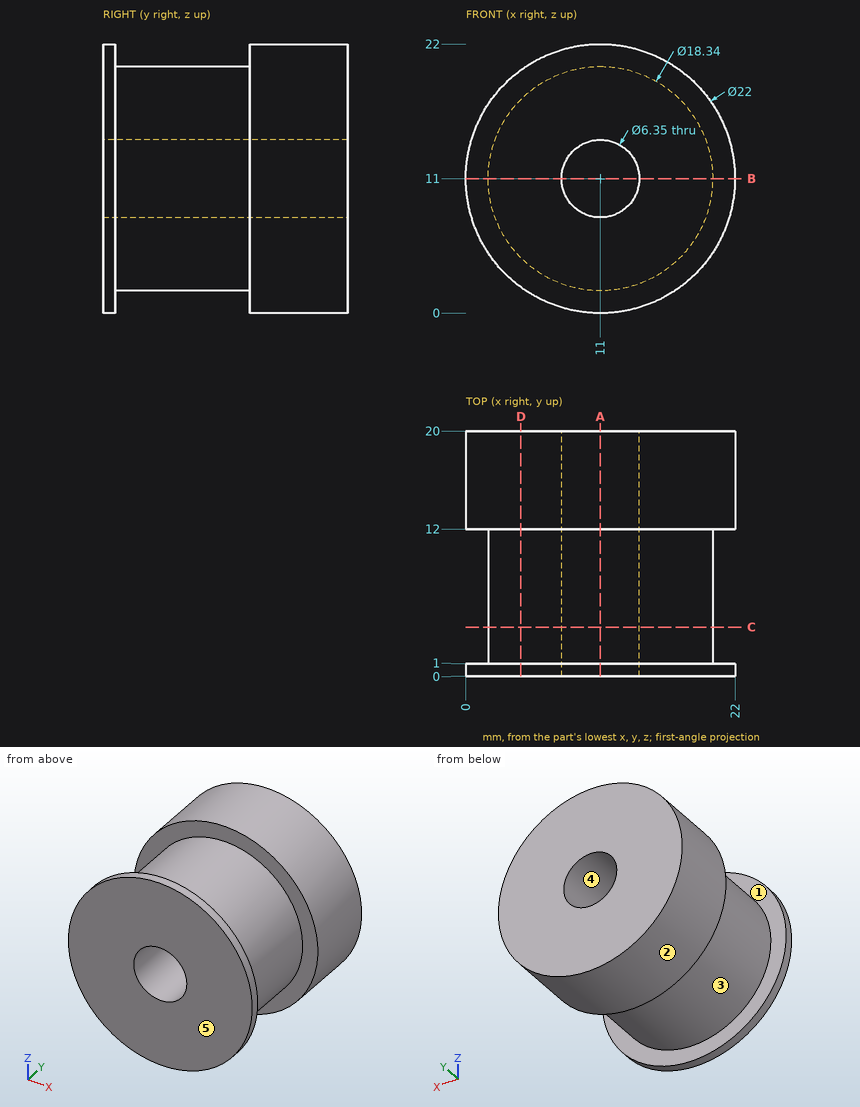
Answer from the drawing. Dimensions are ordinates in mm from the lowest x, y and z of the part. A direction names the side the tool comes from. Give positions to 0.01 mm unless a question says otherwise; leave off trailing zeros. Order: outer loops, then holes, each group sorted by start corner. A loop starts at its lowest first (then second) coordinate and runs counter-clockwise, first axis right, second up.
(1) Find section C-C (y = 4). Give the vertices of the cut face in (x, z) (3 decimals).
(2) Find section A-A (x = 11). Give the vertices of the cut face in (y, z) (3 decimals).
(3) For a pull along X with two mould halves and no side action, classify the marked faces 3, 4 and 5 as released by +X, released by -X, zero draft, split by the parting line, or undercut.
(4) For the marked faces 1 and 2, determine the directions among +Z, -Z, +X, -X, +Y, -Y from which every point of the face is accessible in a straight line to the end or side of a thin tool.
(5) Find section D-D (x = 4.5). Give the vertices of the cut face in (y, z), plus the area to 3 significant figures.
(6) Given pin 1 (10 mm diameter, centred on x = 11, z = 11, fed in from -Y); pin 2 (4 mm diameter, centred on y = 5, z = 5.5, fed in from +X); pin 3 (1.5 mm diameter, centred on x = 14, y = 6.5, fed in from +Z); pin 4 (10 mm diameter, centred on x = 18, y = 13.5, fed in from -Z), each flat-ended and moving along its own axis, determine where each tip first touches the part or whether it passes through.
(7) Find section B-B (z = 11). Give the vertices of the cut face in (x, y) (3 decimals), plus the area to 3 significant figures.
(8) Straight lines are drawn through the part: L1, parallel to X at y = 14.25, z = 11 (3 decimals); L2, parallel to Y at x = 4.75, z = 18.5; L3, parallel to X at y = 4.25, z = 11 (3 decimals). For each, find the intervals that lie inside material, in ascending order.
Result sheet:
1. outline: circle Ø18.34 at (11, 11); hole circle Ø6.35 at (11, 11)
2. outline: (0, 0) - (1, 0) - (1, 1.83) - (12, 1.83) - (12, 0) - (20, 0) - (20, 7.825) - (0, 7.825) - close; (0, 14.175) - (20, 14.175) - (20, 22) - (12, 22) - (12, 20.17) - (1, 20.17) - (1, 22) - (0, 22) - close
3. face 3: split by the parting line
3. face 4: undercut
3. face 5: zero draft
4. face 1: none
4. face 2: +Y, -Y
5. outline: (0, 2.13) - (1, 2.13) - (1, 4.53) - (12, 4.53) - (12, 2.13) - (20, 2.13) - (20, 19.87) - (12, 19.87) - (12, 17.47) - (1, 17.47) - (1, 19.87) - (0, 19.87) - close
5. area: 302 mm2
6. pin 1: stops at y = 0
6. pin 2: stops at x = 19.48
6. pin 3: stops at z = 19.89
6. pin 4: stops at z = 0.18
7. outline: (0, 0) - (7.825, 0) - (7.825, 20) - (0, 20) - (0, 12) - (1.83, 12) - (1.83, 1) - (0, 1) - close; (14.175, 0) - (22, 0) - (22, 1) - (20.17, 1) - (20.17, 12) - (22, 12) - (22, 20) - (14.175, 20) - close
7. area: 273 mm2
8. L1: x = 0 to 7.825, 14.175 to 22
8. L2: y = 0 to 1, 12 to 20
8. L3: x = 1.83 to 7.825, 14.175 to 20.17
